```python
from build123d import *

# Parameters (mm, degrees)
SKETCH_1_R          = 1.6
SKETCH_1_R_2        = 6.05
EXTRUDE_1_DEPTH     = 11
SKETCH_2_R          = 1.65
CUT_EXTRUDE_3_DEPTH = 24.270152556
SKETCH_3_R          = 1.65
CUT_EXTRUDE_4_DEPTH = 24.270152604


with BuildPart() as part:
    # ｽｹｯﾁ1 → ﾎﾞｽ - 押し出し1 (new body)
    with BuildSketch(Plane.XY):
        with BuildLine():
            Line((1, 12.459935794), (0.75, 14.5))
            Line((0.75, 14.5), (-0.75, 14.5))
            Line((-0.75, 14.5), (-1, 12.459935794))
            ThreePointArc((-1, 12.459935794), (-1.955430813, 12.346104257), (-2.899275393, 12.159120124))
            Line((-2.899275393, 12.159120124), (-3.767454031, 14.022082232))
            Line((-3.767454031, 14.022082232), (-5.194038806, 13.55855674))
            Line((-5.194038806, 13.55855674), (-4.801388426, 11.541086135))
            ThreePointArc((-4.801388426, 11.541086135), (-5.674881247, 11.137581552), (-6.51474951, 10.668085059))
            Line((-6.51474951, 10.668085059), (-7.916123412, 12.171585358))
            Line((-7.916123412, 12.171585358), (-9.129648904, 11.289907479))
            Line((-9.129648904, 11.289907479), (-8.132783499, 9.492514554))
            ThreePointArc((-8.132783499, 9.492514554), (-8.838834765, 8.838834765), (-9.492514554, 8.132783499))
            Line((-9.492514554, 8.132783499), (-11.289907479, 9.129648904))
            Line((-11.289907479, 9.129648904), (-12.171585358, 7.916123412))
            Line((-12.171585358, 7.916123412), (-10.668085059, 6.51474951))
            ThreePointArc((-10.668085059, 6.51474951), (-11.137581552, 5.674881247), (-11.541086135, 4.801388426))
            Line((-11.541086135, 4.801388426), (-13.55855674, 5.194038806))
            Line((-13.55855674, 5.194038806), (-14.022082232, 3.767454031))
            Line((-14.022082232, 3.767454031), (-12.159120124, 2.899275393))
            ThreePointArc((-12.159120124, 2.899275393), (-12.346104257, 1.955430813), (-12.459935794, 1))
            Line((-12.459935794, 1), (-14.5, 0.75))
            Line((-14.5, 0.75), (-14.5, -0.75))
            Line((-14.5, -0.75), (-12.459935794, -1))
            ThreePointArc((-12.459935794, -1), (-12.346104257, -1.955430813), (-12.159120124, -2.899275393))
            Line((-12.159120124, -2.899275393), (-14.022082232, -3.767454031))
            Line((-14.022082232, -3.767454031), (-13.55855674, -5.194038806))
            Line((-13.55855674, -5.194038806), (-11.541086135, -4.801388426))
            ThreePointArc((-11.541086135, -4.801388426), (-11.137581552, -5.674881247), (-10.668085059, -6.51474951))
            Line((-10.668085059, -6.51474951), (-12.171585358, -7.916123412))
            Line((-12.171585358, -7.916123412), (-11.289907479, -9.129648904))
            Line((-11.289907479, -9.129648904), (-9.492514554, -8.132783499))
            ThreePointArc((-9.492514554, -8.132783499), (-8.838834765, -8.838834765), (-8.132783499, -9.492514554))
            Line((-8.132783499, -9.492514554), (-9.129648904, -11.289907479))
            Line((-9.129648904, -11.289907479), (-7.916123412, -12.171585358))
            Line((-7.916123412, -12.171585358), (-6.51474951, -10.668085059))
            ThreePointArc((-6.51474951, -10.668085059), (-5.674881247, -11.137581552), (-4.801388426, -11.541086135))
            Line((-4.801388426, -11.541086135), (-5.194038806, -13.55855674))
            Line((-5.194038806, -13.55855674), (-3.767454031, -14.022082232))
            Line((-3.767454031, -14.022082232), (-2.899275393, -12.159120124))
            ThreePointArc((-2.899275393, -12.159120124), (-1.955430813, -12.346104257), (-1, -12.459935794))
            Line((-1, -12.459935794), (-0.75, -14.5))
            Line((-0.75, -14.5), (0.75, -14.5))
            Line((0.75, -14.5), (1, -12.459935794))
            ThreePointArc((1, -12.459935794), (1.955430813, -12.346104257), (2.899275393, -12.159120124))
            Line((2.899275393, -12.159120124), (3.767454031, -14.022082232))
            Line((3.767454031, -14.022082232), (5.194038806, -13.55855674))
            Line((5.194038806, -13.55855674), (4.801388426, -11.541086135))
            ThreePointArc((4.801388426, -11.541086135), (5.674881247, -11.137581552), (6.51474951, -10.668085059))
            Line((6.51474951, -10.668085059), (7.916123412, -12.171585358))
            Line((7.916123412, -12.171585358), (9.129648904, -11.289907479))
            Line((9.129648904, -11.289907479), (8.132783499, -9.492514554))
            ThreePointArc((8.132783499, -9.492514554), (8.838834765, -8.838834765), (9.492514554, -8.132783499))
            Line((9.492514554, -8.132783499), (11.289907479, -9.129648904))
            Line((11.289907479, -9.129648904), (12.171585358, -7.916123412))
            Line((12.171585358, -7.916123412), (10.668085059, -6.51474951))
            ThreePointArc((10.668085059, -6.51474951), (11.137581552, -5.674881247), (11.541086135, -4.801388426))
            Line((11.541086135, -4.801388426), (13.558556741, -5.194038806))
            Line((13.558556741, -5.194038806), (14.022082232, -3.767454031))
            Line((14.022082232, -3.767454031), (12.159120124, -2.899275393))
            ThreePointArc((12.159120124, -2.899275393), (12.346104257, -1.955430813), (12.459935794, -1))
            Line((12.459935794, -1), (14.5, -0.75))
            Line((14.5, -0.75), (14.5, 0.75))
            Line((14.5, 0.75), (12.459935794, 1))
            ThreePointArc((12.459935794, 1), (12.346104257, 1.955430813), (12.159120124, 2.899275393))
            Line((12.159120124, 2.899275393), (14.022082232, 3.767454031))
            Line((14.022082232, 3.767454031), (13.55855674, 5.194038806))
            Line((13.55855674, 5.194038806), (11.541086135, 4.801388426))
            ThreePointArc((11.541086135, 4.801388426), (11.137581552, 5.674881247), (10.668085059, 6.51474951))
            Line((10.668085059, 6.51474951), (12.171585358, 7.916123412))
            Line((12.171585358, 7.916123412), (11.289907479, 9.129648904))
            Line((11.289907479, 9.129648904), (9.492514554, 8.132783499))
            ThreePointArc((9.492514554, 8.132783499), (8.838834765, 8.838834765), (8.132783499, 9.492514554))
            Line((8.132783499, 9.492514554), (9.129648904, 11.289907479))
            Line((9.129648904, 11.289907479), (7.916123412, 12.171585358))
            Line((7.916123412, 12.171585358), (6.51474951, 10.668085059))
            ThreePointArc((6.51474951, 10.668085059), (5.674881247, 11.137581552), (4.801388426, 11.541086135))
            Line((4.801388426, 11.541086135), (5.194038806, 13.55855674))
            Line((5.194038806, 13.55855674), (3.767454031, 14.022082232))
            Line((3.767454031, 14.022082232), (2.899275393, 12.159120124))
            ThreePointArc((2.899275393, 12.159120124), (1.955430813, 12.346104257), (1, 12.459935794))
        make_face()
        with Locations((-9.25, 0)):
            Circle(SKETCH_1_R, mode=Mode.SUBTRACT)
        with Locations((0, -9.25)):
            Circle(SKETCH_1_R, mode=Mode.SUBTRACT)
        Circle(SKETCH_1_R_2, mode=Mode.SUBTRACT)
        with Locations((9.25, 0)):
            Circle(SKETCH_1_R, mode=Mode.SUBTRACT)
        with Locations((0, 9.25)):
            Circle(SKETCH_1_R, mode=Mode.SUBTRACT)
    extrude(amount=EXTRUDE_1_DEPTH)

    # ｽｹｯﾁ2 → ｶｯﾄ - 押し出し3 (cut, through all)
    with BuildSketch(Plane(origin=(0, 0, 0), x_dir=(0, 0, -1), z_dir=(0.7071067811865464, -0.7071067811865488, 0))):
        with Locations(Location((-5.5, 0, 0), (0, 0, 90))):
            Circle(SKETCH_2_R)
    extrude(amount=-CUT_EXTRUDE_3_DEPTH, mode=Mode.SUBTRACT)

    # ｽｹｯﾁ3 → ｶｯﾄ - 押し出し4 (cut, through all)
    with BuildSketch(Plane(origin=(0, 0, 0), x_dir=(0, 0, -1), z_dir=(-0.7071067811865512, -0.7071067811865439, 0))):
        with Locations(Location((-5.5, 0, 0), (0, 0, 90))):
            Circle(SKETCH_3_R)
    extrude(amount=-CUT_EXTRUDE_4_DEPTH, mode=Mode.SUBTRACT)


solid = part.part
```
The model under review builds one solid part; all positions refer to its coordinate system, in mm. A direction names the side the tool comes from. Round coordinates to 2 decimals unless told otherwise and drop trailing zeros. Order: outer loops, then holes, each group sorted by start corner. A loop starts at its lowest first (then second) coordinate and runs counter-clockwise, first axis right, second up.
(1) Tool access review of faces 1 (the face through (5.663, -11.144, 5.423)), 2 (the face through (11.43, -7.225, 5.423)), 3 (the face through (-14.5, 0, 5)), 4 (the face through (-13.494, -0.873, 5.423)), 5 (the face through (0.877, 13.466, 5.423)): name each direction out of +Z, -Z, +X, -X, +Y, -Y from which nothing blocks a thin tool from reaching the whole face with its end or side.
Working result:
face 1: +Z, -Z
face 2: +Z, -Z, +X
face 3: +Z, -Z, -X, +Y, -Y
face 4: +Z, -Z, -X
face 5: +Z, -Z, +Y
(2) For P1, Ø1.5, axis at y = 2.5, z = 6.5, coming from the -X side; P2, Ø3, axis at x = 3, z = 2, coming from the -Y side; P3, Ø2, axis at y = 9, z = 7.5, coming from the +X side; P4, Ø4, axis at x = -9.25, y = 0, coming from the -Z side, all flat-tipped, find the tip position at first contact; note any pin that passes through.
Working result:
P1: stops at x = -12.91
P2: stops at y = -14.02
P3: stops at x = 12.11
P4: stops at z = 0
(3) Take a section at C-C, the plane y = 7.25. Count the separate pieces of the cut face and the enclosed holes in it, plus the area to 3 significant figures.
Working result:
separate pieces: 1
enclosed holes: 2
area: 228 mm2
(4) Mouldability with a two-part tool opening along X and no side actions: class faces 6 (the face through (-8.51, 11.74, 5.42)), 7 (the face through (5.69, 11.13, 5.42)), 8 (the face through (13.494, 0.873, 5.423)), 9 (the face through (-1.94, 12.35, 5.42)) as released by +X, released by -X, zero draft, split by the parting line, or undercut.
Working result:
face 6: released by -X
face 7: undercut
face 8: released by +X
face 9: undercut
(5) Wall thickness on L1, parallel to Y at x = 0, z = 9; L2, parallel to Y at x = 9, z = 4.25; L3, parallel to X at y = 6.5, z = 5.5: over which ranges is each line inside the solid? List them lowest first.
Working result:
L1: y = -14.5 to -10.85, -7.65 to -6.05, 6.05 to 7.65, 10.85 to 14.5
L2: y = -11.38 to -11.06, -8.67 to -1.58, 1.58 to 7.48, 11.06 to 11.38
L3: x = -10.68 to -8.83, -4.17 to 4.17, 8.83 to 10.68
(6) Take a section at A-A, the plane y = 0. State the section outline as (x, z) points, plus the area to 4 significant figures.
Working result:
outline: (-14.5, 0) - (-10.85, 0) - (-10.85, 11) - (-14.5, 11) - close; (-7.65, 0) - (-6.05, 0) - (-6.05, 11) - (-7.65, 11) - close; (6.05, 0) - (7.65, 0) - (7.65, 11) - (6.05, 11) - close; (10.85, 0) - (14.5, 0) - (14.5, 11) - (10.85, 11) - close
area: 115.5 mm2
